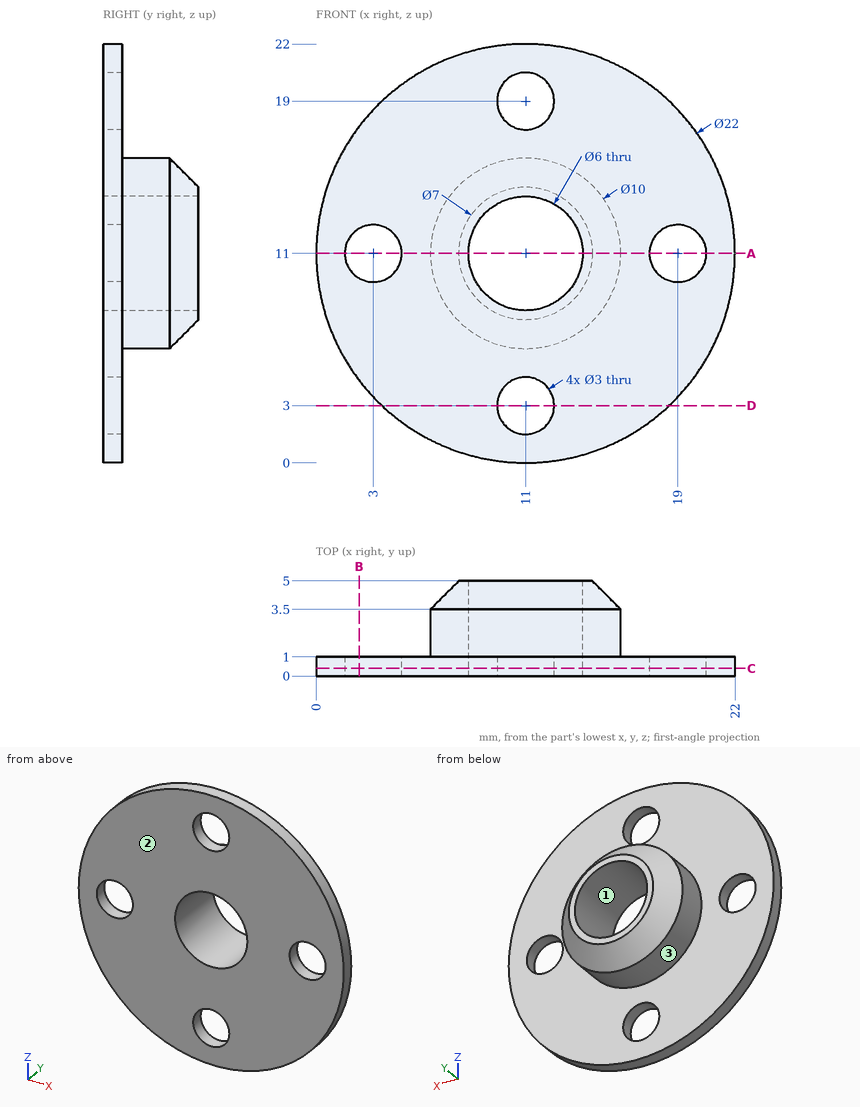
Job drawing, mm, ordinate dimensions from the low corner. One solid piece. Coordinates: 2 decimals unless noted, no trailing zeros. Loops run counter-clockwise (first coordinate to the right, second up) from the corner with the lowest first, then second, coordinate; pieces in that order, holes last. Notation, with made-up numbers: (-30, 18.25) - (9, 18.25) arc R24 cw to (9, 46.25) - close; hole circle Ø6 at (-22, -34). An arc over 180 degrees is marked (long way). Answer as a JSON object with one key per item and string values. Group by question number.
(1) Two-plate mould, pull along Z, no slides. Class the marked faces 1, 2 and 3: released by +Z, released by -Z, zero draft, split by the parting line, or undercut.
(2) Cut at C-C (y = 0.4). Give the cut face in (x, z), then the cut area to 3 significant figures.
(3) Cut at B-B (x = 2.25). Give the cut face in (y, z), then the cut area to 3 significant figures.
(4) Cut at A-A (z = 11). Give the cut face in (x, y), then the cut area to 4 significant figures.
(5) Probe line 1 along X through (y, z) = (0.2, 10); line 2 along Z through (x, y) = (11, 1.5); line 3 along Y through (x, z) = (16, 7.25). List the from-to ranges inside material, lowest first.
(6) Flat gauge pins, fed straight in: pin 1 (1.8 mm diameter, centred on x = 3, z = 11, fed in from +Y); pin 2 (1 mm diameter, centred on y = 2, z = 14.5, fed in from -X); pin 3 (4 mm diameter, centred on x = 20, z = 18.5, fed in from +Y); pin 4 (1 mm diameter, centred on x = 14, z = 6.5, fed in from +Y). Where does each tip first touch, or does it go through?
(7) Cut at D-D (z = 3). Give the cut face in (x, y).
Geometry says:
{
 "1": {"face 1": "undercut", "face 2": "zero draft", "face 3": "split by the parting line"},
 "2": {"outline": "circle Ø22 at (11, 11); hole circle Ø3 at (3, 11); hole circle Ø6 at (11, 11); hole circle Ø3 at (11, 3); hole circle Ø3 at (11, 19); hole circle Ø3 at (19, 11)", "area": "324 mm^2"},
 "3": {"outline": "(0, 4.33) - (1, 4.33) - (1, 9.7) - (0, 9.7) - close; (0, 12.3) - (1, 12.3) - (1, 17.67) - (0, 17.67) - close", "area": "10.7 mm^2"},
 "4": {"outline": "(0, 0) - (1.5, 0) - (1.5, 1) - (0, 1) - close; (4.5, 0) - (8, 0) - (8, 5) - (7.5, 5) - (6, 3.5) - (6, 1) - (4.5, 1) - close; (14, 0) - (17.5, 0) - (17.5, 1) - (16, 1) - (16, 3.5) - (14.5, 5) - (14, 5) - close; (20.5, 0) - (22, 0) - (22, 1) - (20.5, 1) - close", "area": "23.75 mm^2"},
 "5": {"line 1": "x = 0.05 to 1.88, 4.12 to 8.17, 13.83 to 17.88, 20.12 to 21.95", "line 2": "z = 6 to 8, 14 to 16", "line 3": "y = 0 to 1"},
 "6": {"pin 1": "passes through", "pin 2": "stops at x = 7", "pin 3": "stops at y = 1", "pin 4": "stops at y = 3.59"},
 "7": {"outline": "(3.45, 0) - (9.5, 0) - (9.5, 1) - (3.45, 1) - close; (12.5, 0) - (18.55, 0) - (18.55, 1) - (12.5, 1) - close"}
}
